For this review, use the dimensioned drawing (mm, ordinates from the lowest corner) and the shaded views. A direction names the side the tool comes from. Coordinates: 2 decimals unless noted, no trailing zeros. Order: outer loops, then holes, each group sorted by start corner. A loop starts at its lowest first (then second) coordinate and runs counter-clockwise, first axis right, second up. Notation, with made-up numbers: M 75.5,79.25 L 119.5,79.25 A23 cw 119.5,90.25 Z; hole C 17,-15 d9. An arc over 180 degrees is marked long. Use CSV: the item, a comma, the result in double quotes.
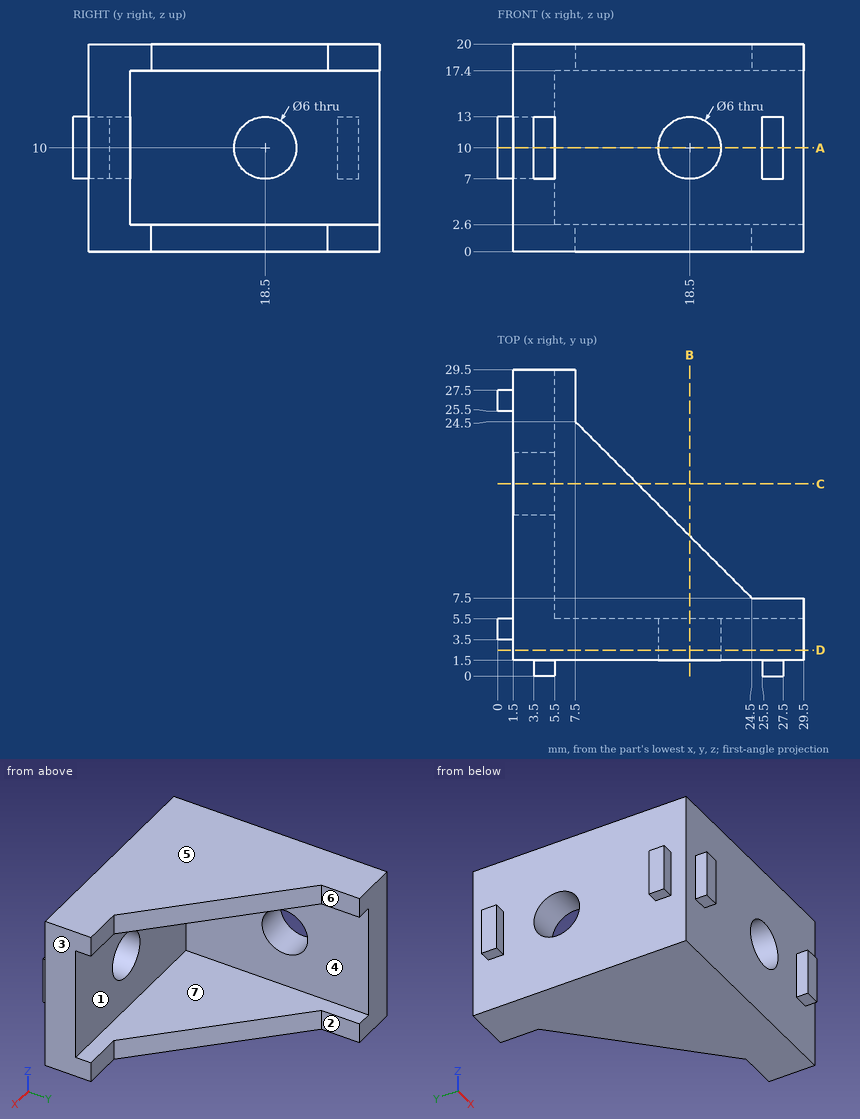
Item 1: Add section D-D on y = 2.5. State the section outline as (x, z) points.
Solutions:
outline,"M 1.5,0 L 29.5,0 L 29.5,20 L 1.5,20 Z; hole C 18.5,10 d6"
Item 2: Add section A-A on z = 10. State how many separate pieces and enclosed holes the cut face has, and give its area (3 significant figures).
Solutions:
separate pieces,"3"
enclosed holes,"0"
area,"172 mm^2"
Item 3: Draft analysis for pull direction Z (two halves, no side actions). For the marked faces 4, 5, 6 and 7, state which applies: released by +Z, released by -Z, zero draft, split by the parting line, or undercut.
Solutions:
face 4,"undercut"
face 5,"released by +Z"
face 6,"zero draft"
face 7,"undercut"
Item 4: Clearance check with flat-ended pins moving along their axes: pin 1 Ø0.5 at (y, z) = (1, 10) entering from -X; pin 2 Ø6 at (y, z) = (18.5, 13) entering from -X; pin 3 Ø10 at (x, z) = (11, 17) entering from -Y; pin 4 Ø1.7 at (x, y) = (5, 1) entering from -Z. State where each tip first meets the part, or that it passes through.
Solutions:
pin 1,"x = 3.5"
pin 2,"x = 1.5"
pin 3,"y = 1.5"
pin 4,"z = 0"
Item 5: Add section B-B on x = 18.5. State the section outline as (y, z) points, and give its area (3 significant figures).
Solutions:
outline,"M 1.5,0 L 13.5,0 L 13.5,2.6 L 5.5,2.6 L 5.5,7 L 1.5,7 Z; M 1.5,13 L 5.5,13 L 5.5,17.4 L 13.5,17.4 L 13.5,20 L 1.5,20 Z"
area,"97.6 mm^2"
Item 6: For the marked faces 1, 2 and 3, list the 3-axis set-ups (+Z, -Z, +X, -X, +Y, -Y) from which the entire face can be reached by the end or side of a thin tool; tool diameter is ignored.
Solutions:
face 1,"+X, +Y"
face 2,"+Z, -Z, +X, +Y"
face 3,"+Z, -Z, +X, +Y, -Y"
Item 7: To check wall thickness, follow line 1 along Z through (x, y) = (7.5, 8.5); line 2 along X through (y, z) = (1, 8.5); line 3 along X through (y, z) = (12.75, 13.75). State the ranges of each line that lie inside material, in increasing order. Write a range as [from, to].
Solutions:
line 1,"[0, 2.6], [17.4, 20]"
line 2,"[3.5, 5.5], [25.5, 27.5]"
line 3,"[1.5, 5.5]"
